Read the model definition and answer for the solid it produces. Units are mm, in the model's axes. A direction names the side the tool comes from. Round coordinates to 2 decimals unless told otherwise and drop trailing zeros. Order: outer loops, then holes, each group sorted by start corner. A loop starts at its lowest first (then second) coordinate and runs counter-clockwise, first axis right, second up. Notation, with made-up numbers: (45, 32.25) -> (80, 32.25) arc R14 ccw to (80, 57.25) -> close; hole circle Ø5 at (32.25, 57.25). An arc over 180 degrees is marked (long way). One line per item, written item: value. Start each with the question number.
1. Section D-D (y = 5.5) is taken. Give the vertices of the cut face in (x, z), then the cut area to 3 significant figures.
2. Section B-B (z = -4) is taken. Give the vertices of the cut face in (x, y), then the cut area to 3 significant figures.
3. For faces 1 (the face through (-7.5, 0, 1)), 2 (the face through (1.05, 0.33, -2.46)), determine the directions among +Z, -Z, +X, -X, +Y, -Y from which every point of the face is accessible in a straight line to the end or side of a thin tool.
4. Section A-A (x = 0) is taken. Give the vertices of the cut face in (y, z), then the cut area to 3 significant figures.
5. A flat-ended cylindrical pin translates along its axis: pin 1 Ø0.7 at (x, y) = (0.5, 0.5) entering from -Z. Find the tip coordinate at first contact, or state that the pin passes through.
6. The mould has two halves that part along X. Classify faces 3 (the face through (-2, 5, 0)), 4 (the face through (7.5, 0, 1)), 5 (the face through (0, 0, 0)): released by +X, released by -X, zero draft, split by the parting line, or undercut.
7. Consider line 1 (Y direction, x = 0, z = -2.05); line 2 (Z direction, x = -0.5, y = -7); line 3 (Z direction, x = 4, y = 0). Determine where each line is inside the solid, lowest interval first.
from build123d import *

# Parameters (mm, degrees)
SKETCH_2_W        = 15
SKETCH_2_H        = 15
EXTRUDE_351_DEPTH = 1.5
SKETCH_3_R        = 3.1
SKETCH_3_R_2      = 1.1
EXTRUDE_479_DEPTH = 5
CHAMFER_1_SIZE    = 2


with BuildPart() as part:
    # Эскиз2 → Extrude 351 (new body)
    with BuildSketch(Plane.XY):
        Rectangle(SKETCH_2_W, SKETCH_2_H)
    extrude(amount=EXTRUDE_351_DEPTH)

    # Эскиз3 → Extrude 479 (add)
    with BuildSketch(Plane.XY):
        Circle(SKETCH_3_R)
        Circle(SKETCH_3_R_2, mode=Mode.SUBTRACT)
    extrude(amount=-EXTRUDE_479_DEPTH)

    # Фаска1
    chamfer_1_edges = [part.edges().sort_by_distance(p)[0] for p in [
        (-3.1, 0, 0),
    ]]
    chamfer(chamfer_1_edges, length=CHAMFER_1_SIZE)


solid = part.part
Answer:
1. outline: (-7.5, 0) -> (7.5, 0) -> (7.5, 1.5) -> (-7.5, 1.5) -> close
1. area: 22.5 mm^2
2. outline: circle Ø6.2 at (0, 0); hole circle Ø2.2 at (0, 0)
2. area: 26.4 mm^2
3. face 1: +Z, -Z, -X, +Y, -Y
3. face 2: -Z
4. outline: (-7.5, 0) -> (-5.1, 0) -> (-3.1, -2) -> (-3.1, -5) -> (-1.1, -5) -> (-1.1, 0) -> (1.1, 0) -> (1.1, -5) -> (3.1, -5) -> (3.1, -2) -> (5.1, 0) -> (7.5, 0) -> (7.5, 1.5) -> (-7.5, 1.5) -> close
4. area: 46.5 mm^2
5. pin 1: z = 0
6. face 3: zero draft
6. face 4: released by +X
6. face 5: undercut
7. line 1: -3.1 to -1.1, 1.1 to 3.1
7. line 2: 0 to 1.5
7. line 3: -1.1 to 1.5
